Check sheet for the modelled part. Datum: model origin and axes. Units: mm. Face numbers are marked on the shaded views. A direction names the side the tool comes from. Give positions to 0.01 mm unless a question says otherwise; leave off trailing zeros. Order: outer loops, then holes, each group sorted by start corner. A loop starts at its lowest first (then second) coordinate and runs counter-clockwise, first axis right, second up.
from build123d import *

# Parameters (mm, degrees)
F1_DEPTH   = 6.35
F3_DEPTH   = 19.05
F3_TAPER   = 10
F4_R       = 6.1659710175
F5_DEPTH   = 31.75
F5_TAPER   = -2
F7_DEPTH   = 25.4
F7_TAPER   = -20
F9_DEPTH   = 38.1
F9_TAPER   = 5
F11_DEPTH  = 38.1
F11_TAPER  = 25
F12_R      = 29.7610911
F13_DEPTH  = 6.35
F13_FACE_R = 29.7610911
F14_DEPTH  = 44.45
F14_TAPER  = -5
F15_DEPTH  = 6.35
F15_FACE_R = 33.6499621937
F16_DEPTH  = 12.7
F16_TAPER  = 60
F17_DEPTH  = 6.35
F17_FACE_R = 11.6529169376
F18_DEPTH  = 12.7
F18_TAPER  = -30
F19_DEPTH  = 31.75
F20_R      = 22.225
F21_DEPTH  = 19.05
F21_TAPER  = 45
F21_FACE_R = 3.175
F22_DEPTH  = 12.7
F22_TAPER  = 1


with BuildPart() as f1:
    # F0 (on Front) → F1 (new body)
    with BuildSketch(Plane.XZ):
        with BuildLine():
            ThreePointArc((3.199654923, 13.4909659788), (3.175, 12.7), (3.199654923, 11.9090340212))
            Line((3.199654923, 11.9090340212), (3.199654923, 13.4909659788))
        make_face()
        with BuildLine():
            Line((15.362857355, 0), (3.199654923, 0))
            Line((3.199654923, 0), (3.199654923, -11.8987034381))
            ThreePointArc((3.199654923, -11.8987034381), (6.9939953282, -3.6112468657), (15.362857355, 0))
        make_face()
        with BuildLine():
            ThreePointArc((16.2371763723, 0.0051652915), (24.9824046777, -3.8383881517), (28.575, -12.6896694169))
            Line((28.575, -12.6896694169), (28.575, 12.7))
            ThreePointArc((28.575, 12.7), (24.9824046777, 3.8487187348), (16.2371763723, 0.0051652915))
        make_face()
        with BuildLine():
            Line((3.199654923, 11.9090340212), (3.199654923, 0))
            Line((3.199654923, 0), (15.362857355, 0))
            ThreePointArc((15.362857355, 0), (15.4378328626, 0.0028041361), (15.5128236277, 0.0051652915))
            ThreePointArc((15.5128236277, 0.0051652915), (7.0477827676, 3.5692696934), (3.199654923, 11.9090340212))
        make_face()
        with BuildLine():
            Line((15.875, 0), (15.362857355, 0))
            ThreePointArc((15.362857355, 0), (6.9939953282, -3.6112468657), (3.199654923, -11.8987034381))
            ThreePointArc((3.199654923, -11.8987034381), (15.4793249297, -25.3835041897), (28.575, -12.6896694169))
            ThreePointArc((28.575, -12.6896694169), (24.9824046777, -3.8383881517), (16.2371763723, 0.0051652915))
            ThreePointArc((16.2371763723, 0.0051652915), (16.0561066018, 0.0012913885), (15.875, 0))
        make_face()
        with BuildLine():
            Line((3.199654923, 13.4909659788), (3.199654923, 11.9090340212))
            ThreePointArc((3.199654923, 11.9090340212), (7.0477827676, 3.5692696934), (15.5128236277, 0.0051652915))
            ThreePointArc((15.5128236277, 0.0051652915), (15.6938933982, 0.0090391945), (15.875, 0.0103305831))
            ThreePointArc((15.875, 0.0103305831), (16.0561066018, 0.0090391945), (16.2371763723, 0.0051652915))
            ThreePointArc((16.2371763723, 0.0051652915), (24.9824046777, 3.8487187348), (28.575, 12.7))
            ThreePointArc((28.575, 12.7), (16.2706750703, 25.3938347728), (3.199654923, 13.4909659788))
        make_face()
    extrude(amount=F1_DEPTH)

    # F2 (on face) → F3, piece 2 (join)
    with BuildSketch(Plane.XZ.offset(6.35)):
        Polygon((15.875, -12.6896694169), (25.4, -12.6896694169), (25.4, 12.7103305831), (6.35, 12.7103305831), (6.35, -12.6896694169), align=None)
    extrude(amount=F3_DEPTH, taper=F3_TAPER)

    # F4 (on face) → F5, piece 2 (join)
    with BuildSketch(Plane.XZ.offset(25.4)):
        with Locations((15.875, 0.0103305831)):
            Circle(F4_R)
    extrude(amount=F5_DEPTH, taper=F5_TAPER)



with BuildPart() as f1b:
    # F0 (on Front) → F1, piece 2 (new body)
    with BuildSketch(Plane.XZ):
        with BuildLine():
            Line((-3.199654923, 13.4909659788), (-3.199654923, 11.9090340212))
            ThreePointArc((-3.199654923, 11.9090340212), (-3.1811652272, 12.3043249297), (-3.175, 12.7))
            ThreePointArc((-3.175, 12.7), (-3.1811652272, 13.0956750703), (-3.199654923, 13.4909659788))
        make_face()
        with BuildLine():
            ThreePointArc((-15.5128236277, 0.0051652915), (-7.0477827676, -3.5589391103), (-3.199654923, -11.8987034381))
            Line((-3.199654923, -11.8987034381), (-3.199654923, 11.9090340212))
            ThreePointArc((-3.199654923, 11.9090340212), (-7.0477827676, 3.5692696934), (-15.5128236277, 0.0051652915))
        make_face()
        with BuildLine():
            ThreePointArc((-16.2371763723, 0.0051652915), (-15.875, 0.0103305831), (-15.5128236277, 0.0051652915))
            ThreePointArc((-15.5128236277, 0.0051652915), (-7.0477827676, 3.5692696934), (-3.199654923, 11.9090340212))
            Line((-3.199654923, 11.9090340212), (-3.199654923, 13.4909659788))
            ThreePointArc((-3.199654923, 13.4909659788), (-16.2706750703, 25.3938347728), (-28.575, 12.7))
            ThreePointArc((-28.575, 12.7), (-24.9824046777, 3.8487187348), (-16.2371763723, 0.0051652915))
        make_face()
        with BuildLine():
            ThreePointArc((-28.575, -12.6896694169), (-15.875, -25.3896694169), (-3.175, -12.6896694169))
            ThreePointArc((-3.175, -12.6896694169), (-3.1811652272, -12.2939943467), (-3.199654923, -11.8987034381))
            ThreePointArc((-3.199654923, -11.8987034381), (-7.0477827676, -3.5589391103), (-15.5128236277, 0.0051652915))
            ThreePointArc((-15.5128236277, 0.0051652915), (-15.875, 0), (-16.2371763723, 0.0051652915))
            ThreePointArc((-16.2371763723, 0.0051652915), (-24.9824046777, -3.8383881517), (-28.575, -12.6896694169))
        make_face()
        with BuildLine():
            Line((-28.575, 12.7), (-28.575, -12.6896694169))
            ThreePointArc((-28.575, -12.6896694169), (-24.9824046777, -3.8383881517), (-16.2371763723, 0.0051652915))
            ThreePointArc((-16.2371763723, 0.0051652915), (-24.9824046777, 3.8487187348), (-28.575, 12.7))
        make_face()
    extrude(amount=F1_DEPTH)

    # F2 (on face) → F3 (join)
    with BuildSketch(Plane.XZ.offset(6.35)):
        Polygon((-25.4, -12.6896694169), (-15.875, -12.6896694169), (-6.35, -12.6896694169), (-6.35, 12.7103305831), (-25.4, 12.7103305831), align=None)
    extrude(amount=F3_DEPTH, taper=F3_TAPER)

    # F4 (on face) → F5 (join)
    with BuildSketch(Plane.XZ.offset(25.4)):
        with Locations((-15.875, 0.0103305831)):
            Circle(F4_R)
    extrude(amount=F5_DEPTH, taper=F5_TAPER)


with BuildPart() as f1_1:
    add(f1.part)

    add(f1b.part)  # F7 merges F1b
    # F6 (on face) → F7 (join)
    with BuildSketch(Plane.XZ.offset(57.15)):
        Polygon((-8.6003018862, -7.5993465171), (-8.6003018862, 0), (-8.5894809611, 7.6199923168), (-23.1605484229, 7.6406842576), (-23.1496981138, 0), (-23.1388771887, -7.6199923168), align=None)
        Polygon((8.5894809611, 7.6199923168), (8.6003018862, 0), (8.6003018862, -7.5993465171), (23.1388771887, -7.6199923168), (23.1496981138, 0), (23.1605484229, 7.6406842576), align=None)
    extrude(amount=F7_DEPTH, taper=F7_TAPER)

    # F8 (on face) → F9 (join)
    with BuildSketch(Plane.XZ.offset(82.55)):
        Polygon((32.4185487065, 16.8986845412), (-32.4185487065, 16.8986845412), (-32.370583502, -16.8779552611), (32.370583502, -16.8779552611), align=None)
    extrude(amount=F9_DEPTH, taper=F9_TAPER)

    # F10 (on face) → F11 (join)
    with BuildSketch(Plane.XZ.offset(120.65)):
        with BuildLine():
            ThreePointArc((25.711790805, -13.5446371807), (28.2114240531, -6.9763124682), (29.061200642, 0))
            ThreePointArc((29.061200642, 0), (28.2086089518, 6.9876865813), (25.7008602101, 13.5653664608))
            Line((25.7008602101, 13.5653664608), (-25.7008602101, 13.5653664608))
            ThreePointArc((-25.7008602101, 13.5653664608), (-28.2135633586, 6.9676556579), (-29.0611713394, -0.0412690571))
            ThreePointArc((-29.0611713394, -0.0412690571), (-28.2064635002, -6.9963418704), (-25.711790805, -13.5446371807))
            Line((-25.711790805, -13.5446371807), (25.711790805, -13.5446371807))
        make_face()
        with BuildLine():
            ThreePointArc((-25.711790805, -13.5446371807), (0, -29.061200642), (25.711790805, -13.5446371807))
            Line((25.711790805, -13.5446371807), (-25.711790805, -13.5446371807))
        make_face()
        with BuildLine():
            Line((-25.7008602101, 13.5653664608), (25.7008602101, 13.5653664608))
            ThreePointArc((25.7008602101, 13.5653664608), (0, 29.061200642), (-25.7008602101, 13.5653664608))
        make_face()
    extrude(amount=-F11_DEPTH, taper=F11_TAPER)

    # F12 (on face) → F13 (join)
    with BuildSketch(Plane.XZ.offset(120.65)):
        Circle(F12_R)
    extrude(amount=F13_DEPTH)

    # F13_face (on face) → F14 (join)
    with BuildSketch(Plane.XZ.offset(127)):
        Circle(F13_FACE_R)
    extrude(amount=F14_DEPTH, taper=F14_TAPER)

    # F15 (add): a face of the model
    f15_faces = [f1_1.faces().sort_by_distance(p)[0] for p in [
        (0, -171.45, 0),
    ]]
    extrude(f15_faces, amount=F15_DEPTH)

    # F15_face (on face) → F16 (join)
    with BuildSketch(Plane.XZ.offset(177.8)):
        Circle(F15_FACE_R)
    extrude(amount=F16_DEPTH, taper=F16_TAPER)

    # F17 (add): a face of the model
    f17_faces = [f1_1.faces().sort_by_distance(p)[0] for p in [
        (0, -190.5, 0),
    ]]
    extrude(f17_faces, amount=F17_DEPTH)

    # F17_face (on face) → F18 (join)
    with BuildSketch(Plane.XZ.offset(196.85)):
        Circle(F17_FACE_R)
    extrude(amount=F18_DEPTH, taper=F18_TAPER)

    # F19 (add): a face of the model
    f19_faces = [f1_1.faces().sort_by_distance(p)[0] for p in [
        (0, -209.55, 0),
    ]]
    extrude(f19_faces, amount=F19_DEPTH)

    # F20 (on face) → F21 (join)
    with BuildSketch(Plane.XZ.offset(241.3)):
        Circle(F20_R)
    extrude(amount=F21_DEPTH, taper=F21_TAPER)

    # F21_face (on face) → F22 (join)
    with BuildSketch(Plane.XZ.offset(260.35)):
        Circle(F21_FACE_R)
    extrude(amount=F22_DEPTH, taper=F22_TAPER)


solid = f1_1.part
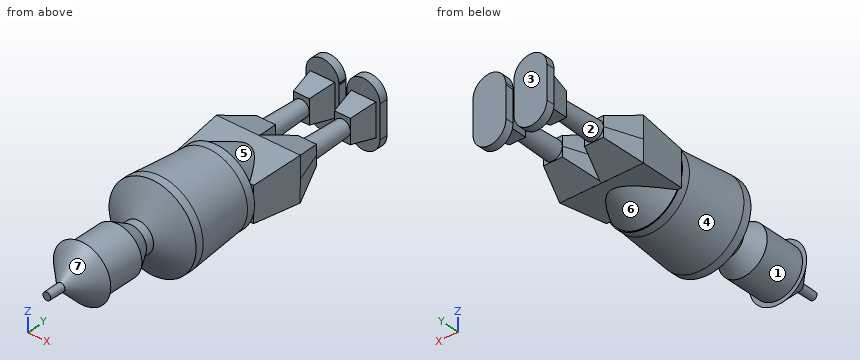
1) Draft check along X on the marked faces 1, 2 and 3. Enter one of: +X half, -X half, draft (parallel to the pull), parting line (faces both ways), or undercut.
Recorded:
face 1: parting line
face 2: undercut
face 3: draft
2) Depth check by flat-ended pin: pin 1 Ø5 at (y, z) = (-4, -4.5) entering from -X (3 decimals); pin 2 Ø7.5 at (x, z) = (17.5, -8) entering from -Y; pin 3 Ø5 at (y, z) = (-125, 18) entering from -X. Enter the tip coordinate at first touch or a pass-through.
Recorded:
pin 1: stops at x = -28.575
pin 2: stops at y = -248.03
pin 3: stops at x = -25.41
3) Section check C-C, the plane y = -137. Record the cut outline in (x, z).
Recorded:
outline: circle Ø61.27 at (0, 0)
4) Material ranges on L1, parallel to Z at x = -15, y = -212; L2, parallel to Y at x = 21, z = 18; L3, parallel to Z at x = 16.5, y = -230.5, recorded low to high.
Recorded:
L1: z = -11.64 to 11.64
L2: y = -181.26 to -117.64, -6.35 to 0
L3: z = -9.39 to 9.39
5) Section check A-A, the plane y = -230. Record the cut outline in (x, z).
Recorded:
outline: circle Ø37.97 at (0, 0)
6) Section check B-B, the plane y = -45.5. Record the cut outline in (x, z) (3 decimals), then the cut area to 3 significant figures.
Recorded:
outline: circle Ø13.736 at (-15.875, 0.01); circle Ø13.736 at (15.875, 0.01)
area: 296 mm2
7) Set-up check for the marked faces 4, 5, 6 and 7: record each of +Z, -Z, +X, -X, +Y, -Y from which the full face is reachable in a straight line by a thin tool's end or side.
Recorded:
face 4: none
face 5: +Z
face 6: -Z
face 7: -Y
